Source: CAD feature listing. Evaluate the final solid. Frame: model axes, mm. Face numbers are marked on the shaded views. A direction names the side the tool comes from. Coordinates: 2 decimals unless noted, no trailing zeros. Write each loop counter-clockwise with the first axis right and the second up, starting at its lowest first coordinate (ties: lowest second). Pieces come first, ordered by that corner, then holes. Notation, with made-up numbers: M 71.5,69.5 L 126.5,69.5 A27 ccw 126.5,97.5 Z; hole C -37.75,80.25 d8. An arc over 180 degrees is marked long. One line per item, written item: value. Start each with the question number.
Item 1: Cut plane C-C, the plane z = 9.75. Output: boundary loops of the cut face in (x, y), then the cut area to 3 significant figures.
Item 2: Mould query, pull axis Y, two halves, no side actions, for the marked faces 1, 2 and 3. Classes: released by +Y, released by -Y, zero draft, split by the parting line, or undercut.
Item 3: Cut plane B-B, the plane x = 4.96. Output: boundary loops of the cut face in (y, z), then the cut area to 3 significant figures.
Item 4: Cut plane D-D, the plane x = 12.75. Output: boundary loops of the cut face in (y, z), then the cut area to 3 significant figures.
Item 5: Pin query (flat end, axial travel): P1, Ø3, axis at x = 24, y = 2.5, coming from the +Z side; P2, Ø8, axis at x = 21.5, y = -16, coming from the +Z side; P3, Ø1.5, axis at x = 23, z = 10, coming from the +Y side. Return the tip coordinate at first contact, or that it passes through.
Item 6: Ray query, L1, parallel to Y at x = 22.84, z = 5.3; L2, parallel to Y at x = 9, z = 3.25; L3, parallel to X at y = -19, z = 9.5. Return the intervals inside material, ascending. Write a range as from..to.
Item 7: Set-up query: the marked faces 4, 5, 6 and 7. Return all of +Z, -Z, +X, -X, +Y, -Y with unobstructed straight access to the full face (end or side cutting, diameter ignored); none if empty.
Item 8: Cut plane A-A, the plane y = -30.65. Output: boundary loops of the cut face in (x, z), then the cut area to 3 significant figures.
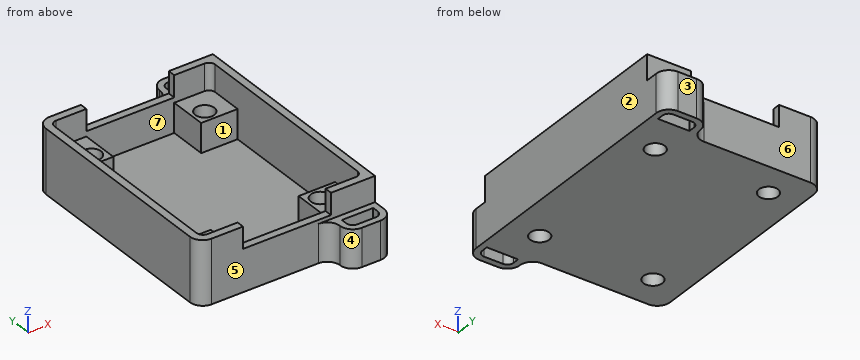
```python
from build123d import *

# Parameters (mm, degrees)
SKIZZE1_W         = 27.8
SKIZZE1_H         = 35.8
EXTRUSION1_DEPTH  = 12
SKIZZE2_W         = 25.4
SKIZZE2_H         = 33.4
EXTRUSION2_DEPTH  = 10.8
SKIZZE3_R         = 1.5
EXTRUSION3_DEPTH  = 10.8
EXTRUSION4_START  = 6.6
SKIZZE4_W         = 5.76
SKIZZE4_H         = 5.95
SKIZZE4_R         = 1.5
EXTRUSION4_DEPTH  = 6.6
SKIZZE5_W         = 13.88
SKIZZE5_H         = 3.4
EXTRUSION5_DEPTH  = 47.887951544
EXTRUSION6_DEPTH  = 2
SKIZZE7_W         = 27.8
SKIZZE7_H         = 35.8
EXTRUSION7_DEPTH  = 2
SKIZZE8_W         = 6.96
SKIZZE8_H         = 6
EXTRUSION8_DEPTH  = 4
SKIZZE9_W         = 4.96
SKIZZE9_H         = 2
EXTRUSION9_DEPTH  = 50.566924456
SKIZZE10_W        = 6.96
SKIZZE10_H        = 4
SKIZZE10_W_2      = 4.96
SKIZZE10_H_2      = 2
EXTRUSION10_DEPTH = 6
RUNDUNG1_R        = 2
RUNDUNG2_R        = 1
RUNDUNG3_R        = 1
SKIZZE11_R        = 1.5
EXTRUSION11_DEPTH = 10


with BuildPart() as part:
    # Skizze1 → Extrusion1 (new body)
    with BuildSketch(Plane.XY):
        with Locations((13.9, -17.9)):
            Rectangle(SKIZZE1_W, SKIZZE1_H)
    extrude(amount=EXTRUSION1_DEPTH)

    # Skizze2 → Extrusion2 (cut)
    with BuildSketch(Plane.XY.offset(12)):
        with Locations((13.9, -17.9)):
            Rectangle(SKIZZE2_W, SKIZZE2_H)
    extrude(amount=-EXTRUSION2_DEPTH, mode=Mode.SUBTRACT)

    # Skizze3 → Extrusion3 (cut)
    with BuildSketch(Plane.XY.offset(1.2)):
        with Locations((22.84, -30.65)):
            Circle(SKIZZE3_R)
        with Locations((4.96, -30.65)):
            Circle(SKIZZE3_R)
        with Locations((22.84, -5.15)):
            Circle(SKIZZE3_R)
        with Locations((4.96, -5.15)):
            Circle(SKIZZE3_R)
    extrude(amount=-EXTRUSION3_DEPTH, mode=Mode.SUBTRACT)

    # Skizze4 → Extrusion4 (add)
    # profile 1 of 4: a face of its own
    with BuildSketch(Plane.XY.offset(1.2).offset(EXTRUSION4_START)):
        with Locations((4.08, -4.175)):
            Rectangle(SKIZZE4_W, SKIZZE4_H)
        with Locations((4.96, -5.15)):
            Circle(SKIZZE4_R, mode=Mode.SUBTRACT)
    # profile 2 of 4: a face of its own
    with BuildSketch(Plane.XY.offset(1.2).offset(EXTRUSION4_START)):
        with Locations((23.72, -4.175)):
            Rectangle(SKIZZE4_W, SKIZZE4_H)
        with Locations((22.84, -5.15)):
            Circle(SKIZZE4_R, mode=Mode.SUBTRACT)
    # profile 3 of 4: a face of its own
    with BuildSketch(Plane.XY.offset(1.2).offset(EXTRUSION4_START)):
        with Locations((23.72, -31.625)):
            Rectangle(SKIZZE4_W, SKIZZE4_H)
        with Locations((22.84, -30.65)):
            Circle(SKIZZE4_R, mode=Mode.SUBTRACT)
    # profile 4 of 4: a face of its own
    with BuildSketch(Plane.XY.offset(1.2).offset(EXTRUSION4_START)):
        with Locations((4.08, -31.625)):
            Rectangle(SKIZZE4_W, SKIZZE4_H)
        with Locations((4.96, -30.65)):
            Circle(SKIZZE4_R, mode=Mode.SUBTRACT)
    extrude(amount=-EXTRUSION4_DEPTH)

    # Skizze5 → Extrusion5 (cut, through all)
    with BuildSketch(Plane(origin=(0, 0, 0), x_dir=(-1, 0, 0), z_dir=(0, 1, 0))):
        with Locations((-13.9, 10.3)):
            Rectangle(SKIZZE5_W, SKIZZE5_H)
    extrude(amount=-EXTRUSION5_DEPTH, mode=Mode.SUBTRACT)

    # Skizze6 → Extrusion6 (add)
    with BuildSketch(Plane.XY.offset(1.2)):
        Polygon((26.6, -1.2), (1.2, -1.2), (1.2, -34.6), (20.84, -34.6), (26.6, -34.6), align=None)
    extrude(amount=EXTRUSION6_DEPTH)

    # Skizze7 → Extrusion7 (cut)
    with BuildSketch(Plane(origin=(0, 0, 0), x_dir=(-1, 0, 0), z_dir=(0, 0, -1))):
        with Locations((-13.9, -17.9)):
            Rectangle(SKIZZE7_W, SKIZZE7_H)
    extrude(amount=-EXTRUSION7_DEPTH, mode=Mode.SUBTRACT)

    # Skizze8 → Extrusion8 (add)
    with BuildSketch(Plane.XZ.offset(35.8)):
        with Locations((24.32, 5)):
            Rectangle(SKIZZE8_W, SKIZZE8_H)
    extrude(amount=EXTRUSION8_DEPTH)

    # Skizze9 → Extrusion9 (cut, through all)
    with BuildSketch(Plane(origin=(0, 0, 2), x_dir=(-1, 0, 0), z_dir=(0, 0, -1))):
        with Locations((-24.32, -37.8)):
            Rectangle(SKIZZE9_W, SKIZZE9_H)
    extrude(amount=-EXTRUSION9_DEPTH, mode=Mode.SUBTRACT)

    # Skizze10 → Extrusion10 (add)
    with BuildSketch(Plane(origin=(0, 0, 2), x_dir=(-1, 0, 0), z_dir=(0, 0, -1))):
        with Locations((-24.32, 2)):
            Rectangle(SKIZZE10_W, SKIZZE10_H)
        with Locations((-24.32, 2)):
            Rectangle(SKIZZE10_W_2, SKIZZE10_H_2, mode=Mode.SUBTRACT)
    extrude(amount=-EXTRUSION10_DEPTH)

    # Rundung1
    rundung1_edges = [part.edges().sort_by_distance(p)[0] for p in [
        (0, 0, 7),
        (0, -35.8, 7),
        (20.84, -39.8, 5),
        (27.8, -39.8, 5),
        (20.84, 4, 5),
        (27.8, 4, 5),
        (20.84, -35.8, 5),
        (20.84, 0, 5),
    ]]
    fillet(rundung1_edges, radius=RUNDUNG1_R - 0.0001)  # a hair under: the kernel refuses the full size

    # Rundung2
    rundung2_edges = [part.edges().sort_by_distance(p)[0] for p in [
        (1.2, -1.2, 9.9),
        (26.6, -1.2, 9.9),
        (26.6, -34.6, 9.9),
        (1.2, -34.6, 9.9),
    ]]
    fillet(rundung2_edges, radius=RUNDUNG2_R)

    # Rundung3
    rundung3_edges = [part.edges().sort_by_distance(p)[0] for p in [
        (26.8, -38.8, 5),
        (21.84, -38.8, 5),
        (21.84, 3, 5),
        (26.8, 3, 5),
    ]]
    fillet(rundung3_edges, radius=RUNDUNG3_R)

    # Skizze11 → Extrusion11 (cut)
    with BuildSketch(Plane.XY.offset(7.8)):
        with Locations((4.96, -5.15)):
            Circle(SKIZZE11_R)
        with Locations((22.84, -5.15)):
            Circle(SKIZZE11_R)
        with Locations((4.96, -30.65)):
            Circle(SKIZZE11_R)
        with Locations((22.84, -30.65)):
            Circle(SKIZZE11_R)
    extrude(amount=-EXTRUSION11_DEPTH, mode=Mode.SUBTRACT)


solid = part.part
```
From the geometry:
1. outline: M 0,-33.8 A2 ccw 2,-35.8 L 6.96,-35.8 L 6.96,-34.6 L 2.2,-34.6 A1 cw 1.2,-33.6 L 1.2,-2.2 A1 cw 2.2,-1.2 L 6.96,-1.2 L 6.96,0 L 2,0 A2 ccw 0,-2 Z; M 20.84,-35.8 L 27.8,-35.8 L 27.8,0 L 20.84,0 L 20.84,-1.2 L 25.6,-1.2 A1 cw 26.6,-2.2 L 26.6,-33.6 A1 cw 25.6,-34.6 L 20.84,-34.6 Z
1. area: 113 mm²
2. face 1: undercut
2. face 2: zero draft
2. face 3: released by +Y
3. outline: M -35.8,2 L -32.15,2 L -32.15,7.8 L -34.6,7.8 L -34.6,12 L -35.8,12 Z; M -29.15,2 L -6.65,2 L -6.65,7.8 L -7.15,7.8 L -7.15,3.2 L -28.65,3.2 L -28.65,7.8 L -29.15,7.8 Z; M -3.65,2 L 0,2 L 0,12 L -1.2,12 L -1.2,7.8 L -3.65,7.8 Z
3. area: 84.0 mm²
4. outline: M -35.8,2 L 0,2 L 0,8.6 L -1.2,8.6 L -1.2,3.2 L -34.6,3.2 L -34.6,8.6 L -35.8,8.6 Z
4. area: 55.9 mm²
5. P1: stops at z = 8
5. P2: stops at z = 3.2
5. P3: stops at y = 0
6. L1: y = -39.8..-38.8, -36.8..-32.15, -29.15..-28.65, -7.15..-6.65, -3.65..1, 3..4
6. L2: y = -35.8..-34.6, -1.2..0
6. L3: x = 0..1.2, 26.6..27.8
7. face 4: +Z, -Z, -X, -Y
7. face 5: +Z, -X, -Y
7. face 6: +Z, -X, +Y
7. face 7: +Z
8. outline: M 0,2 L 3.46,2 L 3.46,7.8 L 1.2,7.8 L 1.2,12 L 0,12 Z; M 6.46,2 L 21.34,2 L 21.34,7.8 L 20.84,7.8 L 20.84,3.2 L 6.96,3.2 L 6.96,7.8 L 6.46,7.8 Z; M 24.34,2 L 27.8,2 L 27.8,12 L 26.6,12 L 26.6,7.8 L 24.34,7.8 Z
8. area: 72.7 mm²
